Geometry: final body of the model. Coordinates: model frame, mm. A direction names the side the tool comes from. Give positions to 0.01 mm unless a question says otherwise; leave off trailing zeros. Order: outer loops, then holes, each group sorted by start corner. A loop starts at its lowest first (then second) coordinate and runs counter-clockwise, first axis right, second up. Notation, with made-up numbers: (-11, 25.25) - (1, 25.25) arc R26 ccw to (1, 52.25) - close; hole circle Ø2 at (24.25, -11.5). An arc over 180 degrees is marked (long way). Put each result on its own line as item: value. Start each with the question number.
1. First-contact query: P1, Ø8, axis at x = 52, y = 1.5, coming from the +Z side. Flat tip, straight axial feed; report the tip coordinate or a pass-through.
2. Ray query, line 1 along Y through (x, z) = (44.5, 0.9); line 2 along X through (y, z) = (14, 1.6); line 3 along Y through (x, z) = (75.05, 1.45). Return the intervals inside material, ascending. Write a range as from..to.
3. Section D-D on z = 1.8. Count the separate pieces of the cut face and the enclosed holes in it, plus the area to 3 significant figures.
4. Section B-B on y = -9. Return the cut outline in (x, z), plus the area to 3 significant figures.
5. Set-up query: faces 1 (the flat face through (36, -3, 0)), 2 (the flat face through (67, 0, 2)). Return all of +Z, -Z, +X, -X, +Y, -Y with unobstructed straight access to the full face (end or side cutting, diameter ignored); none if empty.
6. Mould query, pull axis X, two halves, no side actions, for faces 3 (the flat face through (-3.65, -3, 2)), 4 (the flat face through (67, 14.1, 2)), 5 (the flat face through (36, -3, 4)). Classes: pulls with the +X half, pulls with the -X half, needs draft (parallel to the pull), parting line crosses it, or undercut.
7. Section C-C on x = 28. Return the cut outline in (y, z), plus the area to 3 significant figures.
8. Section A-A on y = -2.95. Return the cut outline in (x, z), plus the area to 3 significant figures.
Autodesk Inventor part; units mm, degrees
ref_plane "YZ Plane" through (0, 0, 0) normal (1, 0, 0) x (0, 1, 0)
ref_plane "XZ Plane" through (0, 0, 0) normal (0, 1, 0) x (-1, 0, 0)
ref_plane "XY Plane" through (0, 0, 0) normal (0, 0, 1) x (1, 0, 0)
sketch "Sketch2" plane through (0, 0, 0) normal (0, 0, 1) x (1, 0, 0)
  line L0 (0, 0) -> (14.1, 0)
  line L1 (14.1, 0) -> (14.1, 14.1)
  line L2 (14.1, 14.1) -> (0, 14.1)
  line L3 (0, 14.1) -> (0, 0)
  line L4 (20, 0) -> (34.1, 0)
  line L5 (34.1, 0) -> (34.1, 14.1)
  line L6 (34.1, 14.1) -> (20, 14.1)
  line L7 (20, 14.1) -> (20, 0)
  line L8 (40, 0) -> (54.1, 0)
  line L9 (54.1, 0) -> (54.1, 14.1)
  line L10 (54.1, 14.1) -> (40, 14.1)
  line L11 (40, 14.1) -> (40, 0)
  line L12 (60, 0) -> (74.1, 0)
  line L13 (74.1, 0) -> (74.1, 14.1)
  line L14 (74.1, 14.1) -> (60, 14.1)
  line L15 (60, 14.1) -> (60, 0)
  line L16 (0, -20) -> (14.1, -20)
  line L17 (14.1, -20) -> (14.1, -5.9)
  line L18 (14.1, -5.9) -> (0, -5.9)
  line L19 (0, -5.9) -> (0, -20)
  line L20 (20, -20) -> (34.1, -20)
  line L21 (34.1, -20) -> (34.1, -5.9)
  line L22 (34.1, -5.9) -> (20, -5.9)
  line L23 (20, -5.9) -> (20, -20)
  line L24 (40, -20) -> (54.1, -20)
  line L25 (54.1, -20) -> (54.1, -5.9)
  line L26 (54.1, -5.9) -> (40, -5.9)
  line L27 (40, -5.9) -> (40, -20)
  line L28 (60, -20) -> (74.1, -20)
  line L29 (74.1, -20) -> (74.1, -5.9)
  line L30 (74.1, -5.9) -> (60, -5.9)
  line L31 (60, -5.9) -> (60, -20)
  line L32 (0.05, 18.05) -> (74.05, 18.05)
  line L33 (78.05, 14.05) -> (78.05, -19.95)
  line L34 (74.05, -23.95) -> (0.05, -23.95)
  line L35 (-3.95, -19.95) -> (-3.95, 14.05)
  arc A0 (0.05, 18.05) -> (-3.95, 14.05) centre (0.05, 14.05) ccw
  arc A1 (-3.95, -19.95) -> (0.05, -23.95) centre (0.05, -19.95) ccw
  arc A2 (74.05, -23.95) -> (78.05, -19.95) centre (74.05, -19.95) ccw
  arc A3 (78.05, 14.05) -> (74.05, 18.05) centre (74.05, 14.05) ccw
  circle A4 centre (-0.95, -2.95) radius 1.15
  circle A5 centre (75.05, -2.95) radius 1.15
  point P0 (-3.95, 18.05)
  point P1 (78.05, -23.95)
  point P2 (78.05, 18.05)
  point P3 (-3.95, -23.95)
  dimension "d0" = 14.1
  dimension "d1" = 14.1
  dimension "d6" = 20
  dimension "d9" = 20
  dimension "d18" = 4
  dimension "d19" = 2.3
  dimension "d20" = 3
  dimension "d22" = 21
  dimension "d23" = 42
  dimension "d24" = 82
  dimension "d25" = 3
  dimension "d26" = 21
  dimension "d27" = 23.95
  dimension "d28" = 38.05
extrude "Extrusion1" add sketch "Sketch2" along normal blind 4
chamfer "Chamfer1" distance 1.5 angle 45 2 edges at (-2.1, -2.95, 4) (73.9, -2.95, 4)
sketch "Sketch3" plane through (0, 0, 4) normal (0, 0, 1) x (1, 0, 0)
  line L0 (0.05, 18.05) -> (74.05, 18.05)
  line L1 (78.05, 14.05) -> (78.05, -19.95)
  line L2 (74.05, -23.95) -> (0.05, -23.95)
  line L3 (-3.95, -19.95) -> (-3.95, 14.05)
  arc A0 (0.05, 18.05) -> (-3.95, 14.05) centre (0.05, 14.05) ccw
  arc A1 (-3.95, -19.95) -> (0.05, -23.95) centre (0.05, -19.95) ccw
  arc A2 (74.05, -23.95) -> (78.05, -19.95) centre (74.05, -19.95) ccw
  arc A3 (78.05, 14.05) -> (74.05, 18.05) centre (74.05, 14.05) ccw
  line L4 (74.05, 17.75) -> (0.05, 17.75)
  arc A4 (0.05, 17.75) -> (-3.65, 14.05) centre (0.05, 14.05) ccw
  line L5 (-3.65, 14.05) -> (-3.65, -19.95)
  arc A5 (-3.65, -19.95) -> (0.05, -23.65) centre (0.05, -19.95) ccw
  line L6 (0.05, -23.65) -> (74.05, -23.65)
  arc A6 (74.05, -23.65) -> (77.75, -19.95) centre (74.05, -19.95) ccw
  line L7 (77.75, -19.95) -> (77.75, 14.05)
  arc A7 (77.75, 14.05) -> (74.05, 17.75) centre (74.05, 14.05) ccw
  point P0 (0, 0)
  dimension "d32" = 4
  dimension "d33" = 0.3
extrude "Extrusion2" cut sketch "Sketch3" against normal blind 10
properties part number "Plate"
Resolved:
1. P1: z = 4
2. line 1: -23.65..-20, -5.9..0, 14.1..17.75
2. line 2: -3.65..0, 14.1..20, 34.1..40, 54.1..60, 74.1..77.75
2. line 3: -23.51..-4.1, -1.8..17.61
3. separate pieces: 1
3. enclosed holes: 10
3. area: 1,760 mm^2
4. outline: (-3.65, 0) - (0, 0) - (0, 4) - (-3.65, 4) - close; (14.1, 0) - (20, 0) - (20, 4) - (14.1, 4) - close; (34.1, 0) - (40, 0) - (40, 4) - (34.1, 4) - close; (54.1, 0) - (60, 0) - (60, 4) - (54.1, 4) - close; (74.1, 0) - (77.75, 0) - (77.75, 4) - (74.1, 4) - close
4. area: 100 mm^2
5. face 1: -Z, +X, -X, +Y, -Y
5. face 2: +Z, -Z
6. face 3: pulls with the -X half
6. face 4: undercut
6. face 5: needs draft
7. outline: (-23.65, 0) - (-20, 0) - (-20, 4) - (-23.65, 4) - close; (-5.9, 0) - (0, 0) - (0, 4) - (-5.9, 4) - close; (14.1, 0) - (17.75, 0) - (17.75, 4) - (14.1, 4) - close
7. area: 52.8 mm^2
8. outline: (-3.65, 0) - (-2.1, 0) - (-2.1, 2.5) - (-3.6, 4) - (-3.65, 4) - close; (0.2, 0) - (73.9, 0) - (73.9, 2.5) - (72.4, 4) - (1.7, 4) - (0.2, 2.5) - close; (76.2, 0) - (77.75, 0) - (77.75, 4) - (77.7, 4) - (76.2, 2.5) - close
8. area: 303 mm^2
